Build history of the part. All positions in model axes, mm. Round coordinates to 2 decimals unless told otherwise and drop trailing zeros. Loops run counter-clockwise (first coordinate to the right, second up) from the corner with the lowest first, then second, coordinate; pieces in that order, holes last. Notation, with made-up numbers: (71.5, 6.5) - (91.5, 6.5) arc R21 ccw to (91.5, 34.5) - close; hole circle Ø7 at (80, 30.25). An arc over 180 degrees is marked (long way). Put each result on its own line as item: value. Start each with the question number.
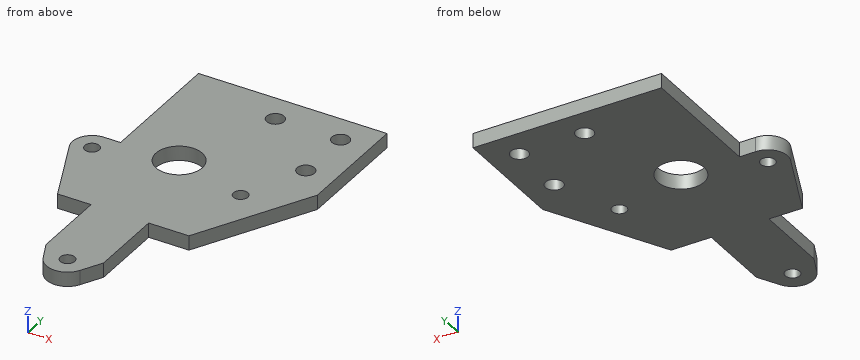
Autodesk Fusion 360 part; units mm, degrees
sketch "Sketch1" plane through (0, 0, 0) normal (0, 0, 1) x (1, 0, 0)
  circle A0 centre (-25.7238, 28.3736) radius 2.5
  circle A1 centre (25.5, 28.3736) radius 2.5
  circle A2 centre (-0.0118, -28.6264) radius 2.5
  line L0 (45, 40) -> (45, 80)
  line L1 (45, 80) -> (25, 80)
  circle A3 centre (35, 50) radius 3
  circle A4 centre (12.5, 70) radius 3
  arc A5 (-6.6169, -31.6214) -> (6.3787, -32.0555) centre (-0.0118, -28.6264) ccw
  line L2 (-9.6692, 1.0232) -> (-9.6692, -24.8899)
  line L3 (10.2145, -24.9071) -> (10.2145, 1)
  line L4 (10.2145, 1) -> (24.0728, 1)
  line L5 (-9.6692, 1.0232) -> (-21.2251, 1.0232)
  line L6 (6.3787, -32.0555) -> (10.2145, -24.9071)
  line L7 (24.0728, 1) -> (45, 40)
  line L8 (-9.6692, -24.8899) -> (-6.6169, -31.6214)
  line L9 (-20, 35.1708) -> (-20, 80)
  line L10 (-20, 80) -> (25, 80)
  line L11 (-21.2251, 1.0232) -> (-31.7762, 25.2695)
  line L12 (-25.47, 35.1708) -> (-20, 35.1708)
  arc A6 (-25.47, 35.1708) -> (-31.7762, 25.2695) centre (-25.7238, 28.3736) ccw
  circle A7 centre (0, 35.5) radius 8
  circle A8 centre (35, 70) radius 3
  point P0 (0, 35.5)
  dimension "d43" = 16
  dimension "d46" = 6
extrude "Extrude5" add sketch "Sketch1" along normal blind 5
Item 1: Drill centre lines: probe 1 along Y at (x, z) = (35, 3.3); probe 2 along X at (y, z) = (70.5, 0.4); probe 3 along X at (y, z) = (-1, 3.7). Where is each one in solid material? Low to high. Write a range as [from, to].
Item 2: Slice it at A-A (y = 70). Give the cut face in (x, z).
Item 3: Slice it at C-C (z = 3.6). Give the cut face in (x, y), plus the area to 3 significant figures.
Item 4: Drop flat-ended pins along their axis: pin 1 Ø1.5 at (y, z) = (-14, 2.5) entering from +X; pin 2 Ø1.5 at (x, z) = (17.5, 2) entering from -Y; pin 3 Ø4 at (x, y) = (23.5, 0.5) entering from +Z. Give the stop position or say it passes through.
Item 5: Slice it at D-D (y = 37.5). Give the cut face in (x, z).
Item 6: Slice it at B-B (x = 12.5). Give the cut face in (y, z).
Computed values:
1. probe 1: y = [21.36, 47], [53, 67], [73, 80]
1. probe 2: x = [-20, 9.54], [15.46, 32.04], [37.96, 45]
1. probe 3: x = [-9.67, 10.21]
2. outline: (-20, 0) - (9.5, 0) - (9.5, 5) - (-20, 5) - close; (15.5, 0) - (32, 0) - (32, 5) - (15.5, 5) - close; (38, 0) - (45, 0) - (45, 5) - (38, 5) - close
3. outline: (-31.78, 25.27) - (-21.23, 1.02) - (-9.67, 1.02) - (-9.67, -24.89) - (-6.62, -31.62) arc R7.25 ccw to (6.38, -32.06) - (10.21, -24.91) - (10.21, 1) - (24.07, 1) - (45, 40) - (45, 80) - (-20, 80) - (-20, 35.17) - (-25.47, 35.17) arc R6.8 ccw to start; hole circle Ø5 at (-25.72, 28.37); hole circle Ø16 at (0, 35.5); hole circle Ø5 at (-0.01, -28.63); hole circle Ø6 at (12.5, 70); hole circle Ø5 at (25.5, 28.37); hole circle Ø6 at (35, 50); hole circle Ø6 at (35, 70)
3. area: 5,320 mm^2
4. pin 1: stops at x = 10.21
4. pin 2: stops at y = 1
4. pin 3: stops at z = 5
5. outline: (-20, 0) - (-7.75, 0) - (-7.75, 5) - (-20, 5) - close; (7.75, 0) - (43.66, 0) - (43.66, 5) - (7.75, 5) - close
6. outline: (1, 0) - (67, 0) - (67, 5) - (1, 5) - close; (73, 0) - (80, 0) - (80, 5) - (73, 5) - close
